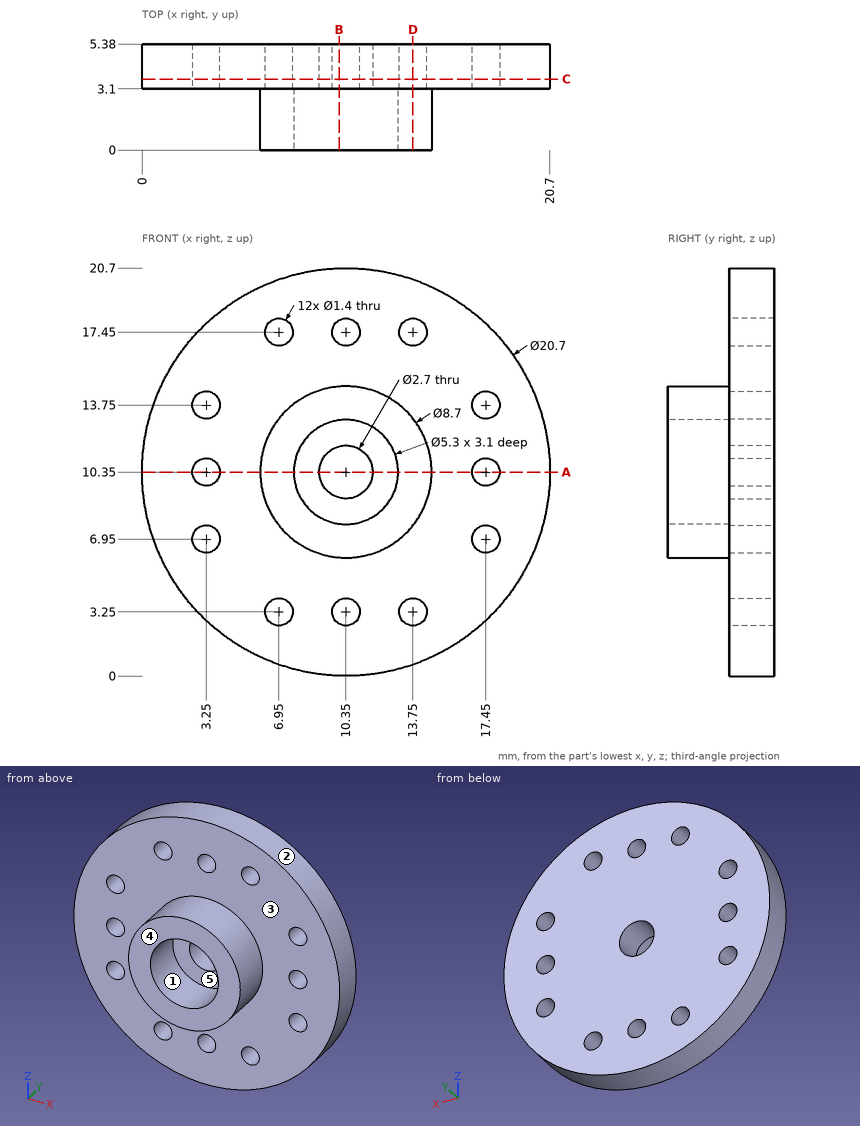
Drawing for the job (mm, zero at the part's lowest x, y, z). A direction names the side the tool comes from. Give positions to 0.01 mm unless a question says otherwise; leave off trailing zeros. Order: outer loops, then holes, each group sorted by start corner. A loop starts at its lowest first (then second) coordinate and runs counter-clockwise, first axis right, second up. Notation, with made-up numbers: (43.25, 85.25) - (74.25, 85.25) arc R21 cw to (74.25, 100.25) - close; hole circle Ø3 at (39, 34). An arc over 180 degrees is marked (long way). Write item = value, one per line. Start each with the question number.
1. Two-plate mould, pull along X, no slides. Class the marked faces 1, 2 and 3: pulls with the +X half, pulls with the -X half, needs draft (parallel to the pull), parting line crosses it, or undercut.
2. Cut at B-B, the plane x = 10. List the corners of the cut face in (y, z).
3. Cut at C-C, the plane y = 3.6. State how many separate pieces and enclosed holes the cut face has, and give its area (3 significant figures).
4. Cut at A-A, the plane z = 10.35. List the corners of the cut face in (x, y).
5. Drop flat-ended pins along their axis: P1, Ø1.5, axis at x = 7, y = 2, coming from the -Z side; P2, Ø1, axis at x = 4, y = 4, coming from the +Z side; P3, Ø1.6, axis at x = 9, z = 11, coming from the -Y side. Give the stop position or say it passes through.
6. Cut at D-D, the plane x = 13.75. List the corners of the cut face in (y, z), and give its area (3 significant figures).
7. Which spindle directions (+Z, -Z, +X, -X, +Y, -Y) get a long thin tool onto all of the face, cutting with end or side? Do the marked faces 4 and 5. Say none if no direction does.
8. Probe line 1 along Z through (x, y) = (10.35, 3.95); line 2 along Z through (x, y) = (13.75, 4.4); line 3 along X through (y, z) = (3.75, 17.5). List the from-to ranges inside material, lowest first.
Taken from the geometry:
q1.face_1 = undercut
q1.face_2 = parting line crosses it
q1.face_3 = needs draft
q2.outline = (0, 6.01) - (3.1, 6.01) - (3.1, 3.86) - (5.38, 3.86) - (5.38, 9.05) - (3.1, 9.05) - (3.1, 7.72) - (0, 7.72) - close; (0, 12.98) - (3.1, 12.98) - (3.1, 11.65) - (5.38, 11.65) - (5.38, 16.84) - (3.1, 16.84) - (3.1, 14.69) - (0, 14.69) - close; (3.1, 0.01) - (5.38, 0.01) - (5.38, 2.64) - (3.1, 2.64) - close; (3.1, 18.06) - (5.38, 18.06) - (5.38, 20.69) - (3.1, 20.69) - close
q3.separate_pieces = 1
q3.enclosed_holes = 13
q3.area = 312 mm²
q4.outline = (0, 3.1) - (2.55, 3.1) - (2.55, 5.38) - (0, 5.38) - close; (3.95, 3.1) - (6, 3.1) - (6, 0) - (7.7, 0) - (7.7, 3.1) - (9, 3.1) - (9, 5.38) - (3.95, 5.38) - close; (11.7, 3.1) - (13, 3.1) - (13, 0) - (14.7, 0) - (14.7, 3.1) - (16.75, 3.1) - (16.75, 5.38) - (11.7, 5.38) - close; (18.15, 3.1) - (20.7, 3.1) - (20.7, 5.38) - (18.15, 5.38) - close
q5.P1 = 6.86
q5.P2 = 18.89
q5.P3 = 3.1
q6.outline = (0, 7.64) - (3.1, 7.64) - (3.1, 3.95) - (5.38, 3.95) - (5.38, 16.75) - (3.1, 16.75) - (3.1, 13.06) - (0, 13.06) - close; (3.1, 0.57) - (5.38, 0.57) - (5.38, 2.55) - (3.1, 2.55) - close; (3.1, 18.15) - (5.38, 18.15) - (5.38, 20.13) - (3.1, 20.13) - close
q6.area = 55.0 mm²
q7.face_4 = +Z, -Z, +X, -X, -Y
q7.face_5 = -Y
q8.line_1 = 0 to 2.55, 3.95 to 9, 11.7 to 16.75, 18.15 to 20.7
q8.line_2 = 0.57 to 2.55, 3.95 to 16.75, 18.15 to 20.13
q8.line_3 = 2.87 to 6.25, 7.65 to 9.65, 11.05 to 13.05, 14.45 to 17.83
